```python
from build123d import *

# Parameters (mm, degrees)
ESQUISSE1_R      = 2.5
EXTRUSION1_DEPTH = 8
ESQUISSE2_R      = 4
EXTRUSION2_DEPTH = 4
ESQUISSE3_R      = 2
EXTRUSION3_DEPTH = 15


with BuildPart() as part:
    # Esquisse1 → Extrusion1 (new body)
    with BuildSketch(Plane.XY):
        Polygon((-20, -20), (-20, 5), (-15, 10), (15, 10), (20, 5), (20, -20), align=None)
        Circle(ESQUISSE1_R, mode=Mode.SUBTRACT)
    extrude(amount=EXTRUSION1_DEPTH)

    # Esquisse2 → Extrusion2 (cut)
    with BuildSketch(Plane.XY.offset(8)):
        Circle(ESQUISSE2_R)
    extrude(amount=-EXTRUSION2_DEPTH, mode=Mode.SUBTRACT)

    # Esquisse3 → Extrusion3 (cut)
    with BuildSketch(Plane.XZ.offset(20)):
        with Locations((-15.5, 4)):
            Circle(ESQUISSE3_R)
        with Locations((15.5, 4)):
            Circle(ESQUISSE3_R)
    extrude(amount=-EXTRUSION3_DEPTH, mode=Mode.SUBTRACT)


solid = part.part
```
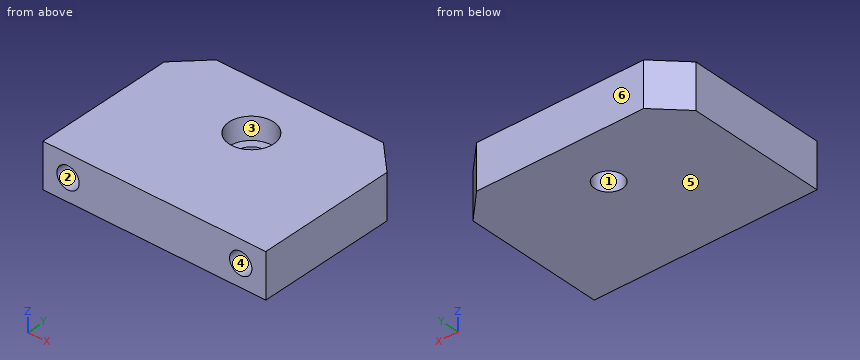
Can you work these out from the model? Positions are in its coordinate system, mm. Face numbers are marked on the shaded views. A direction names the side the tool comes from. Give positions to 0.01 mm unless a question says otherwise; leave off trailing zeros. Order: outer loops, then holes, each group sorted by start corner. A loop starts at its lowest first (then second) coordinate and runs counter-clockwise, first axis right, second up. Notation, with made-up numbers: M -10.5,-33.75 L 26.5,-33.75 A28 ccw 26.5,-6.75 Z; hole C 23,-16.5 d2. An arc over 180 degrees is marked long. One line per item, written item: value.
1) For P1, Ø6.5, axis at x = 0, y = 0.5, coming from the +Z side, with a flat end and sliding along its axis, tell me the tip position at first contact or that it passes through.
Answer sheet:
P1: stops at z = 4
2) Please list where these lines run through material, in increasing order: line 1 along X through (y, z) = (0, 1.9); line 2 along Y through (x, z) = (0, 5.4); line 3 along Z through (x, y) = (15.5, -12.25).
Answer sheet:
line 1: x = -20 to -2.5, 2.5 to 20
line 2: y = -20 to -4, 4 to 10
line 3: z = 0 to 2, 6 to 8
3) I want a section at B-B, the plane x = 0. List the corners of the cut face in (y, z) for me.
Answer sheet:
outline: M -20,0 L -2.5,0 L -2.5,4 L -4,4 L -4,8 L -20,8 Z; M 2.5,0 L 10,0 L 10,8 L 4,8 L 4,4 L 2.5,4 Z
4) I want a section at D-D, the plane x = -15.5. List the corners of the cut face in (y, z) for me, plus the area to 3 significant figures.
Answer sheet:
outline: M -20,0 L 9.5,0 L 9.5,8 L -20,8 L -20,6 L -5,6 L -5,2 L -20,2 Z
area: 176 mm^2
5) On a 3-axis mill with a long thin cutter (end or side, diameter ignored), from which of +Z, -Z, +X, -X, +Y, -Y can I reach the whole of each face in a straight line? I mean the marked faces 1, 2 and 3. Say none if no direction works.
Answer sheet:
face 1: +Z, -Z
face 2: -Y
face 3: +Z
6) We'd pull the mould along Z, two halves only. Please class the marked faces 4, 5 and 6: released by +Z, released by -Z, zero draft, split by the parting line, or undercut.
Answer sheet:
face 4: undercut
face 5: released by -Z
face 6: zero draft
7) I want a section at C-C, the plane z = 1.5. List the corners of the cut face in (x, y) for me.
Answer sheet:
outline: M -20,-20 L 20,-20 L 20,5 L 15,10 L -15,10 L -20,5 Z; hole C 0,0 d5
8) I want a section at A-A, the plane y = 0. List the corners of the cut face in (x, z) for me.
Answer sheet:
outline: M -20,0 L -2.5,0 L -2.5,4 L -4,4 L -4,8 L -20,8 Z; M 2.5,0 L 20,0 L 20,8 L 4,8 L 4,4 L 2.5,4 Z
